The model under review builds one solid part; all positions refer to its coordinate system, in mm. Face numbers are marked on the shaded views. A direction names the side the tool comes from. Round coordinates to 2 decimals unless told otherwise and drop trailing zeros. Order: outer loops, then holes, each group sorted by start corner. A loop starts at its lowest first (then second) coordinate and runs counter-clockwise, first axis right, second up. Notation, with made-up numbers: M 83.5,-38 L 137.5,-38 A20 cw 137.5,-3 Z; hole C 72,57.25 d1. An arc over 180 degrees is marked long. Answer as CSV lines item,"result". Start each with the question number.
from build123d import *

# Parameters (mm, degrees)
F0_W     = 13
F0_H     = 13
F1_DEPTH = 70
F2_R     = 2
F3_R     = 5.25
F4_DEPTH = 30


with BuildPart() as f1:
    # F0 (on Top) → F1 (new body)
    with BuildSketch(Plane.XY):
        Rectangle(F0_W, F0_H)
    extrude(amount=F1_DEPTH)

    # F2
    f2_edges = [f1.edges().sort_by_distance(p)[0] for p in [
        (0, 6.5, 70),
        (-6.5, 0, 70),
        (0, -6.5, 70),
        (6.5, 0, 70),
    ]]
    fillet(f2_edges, radius=F2_R)

    # F3 (on face) → F4 (join)
    with BuildSketch(Plane.XZ.offset(6.5)):
        with Locations((0, 61.068749)):
            Circle(F3_R)
    extrude(amount=F4_DEPTH)


solid = f1.part
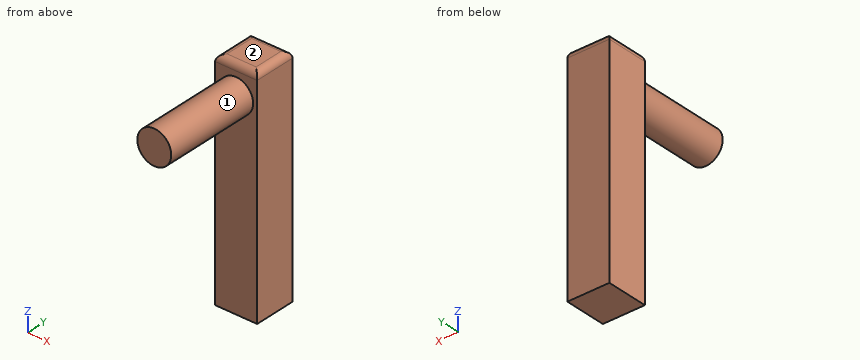
Item 1: Tool access review of the marked faces 1 and 2: name each direction out of +Z, -Z, +X, -X, +Y, -Y from which nothing blocks a thin tool from reaching the whole face with its end or side.
Item 2: Consider section C-C (y = -24.5). State the section outline as (x, z) points, and give its area (3 significant figures).
Item 3: Wall thickness on probe 1 along Y at (x, z) = (3.75, 54.5); probe 2 along Z at (x, y) = (4.75, 0); probe 3 along Z at (x, y) = (5.25, 2): over which ranges is each line inside the solid? List them lowest first. Write a range as [from, to].
Item 4: Consider section A-A (x = 0). State the section outline as (y, z) points, and give its area (3 significant figures).
Item 5: For pin 1 (1.5 mm diameter, centred on x = 0.5, y = -12, fed in from -Z); pin 2 (4 mm diameter, centred on x = 0, z = 37, fed in from -Y); pin 3 (10 mm diameter, centred on y = -10.5, z = 28.5, fed in from +X); pin 4 (4 mm diameter, centred on y = -9.5, z = 62.5, fed in from -X), all flat-tipped, find the tip position at first contact; note any pin that passes through.
Item 6: Consider section B-B (z = 5). State the section outline as (x, y) points, and give its area (3 significant figures).
Reported:
1,face 1,"-Y"
1,face 2,"+Z, +X, -X, +Y, -Y"
2,outline,"C 0,61.07 d10.5"
2,area,"86.6 mm²"
3,probe 1,"y = [-6.5, 6.5]"
3,probe 2,"z = [0, 69.98]"
3,probe 3,"z = [0, 69.85]"
4,outline,"M -36.5,55.82 L -6.5,55.82 L -6.5,0 L 6.5,0 L 6.5,68 A2 ccw 4.5,70 L -4.5,70 A2 ccw -6.5,68 L -6.5,66.32 L -36.5,66.32 Z"
4,area,"1,220 mm²"
5,pin 1,"stops at z = 55.82"
5,pin 2,"stops at y = -6.5"
5,pin 3,"stops at x = 6.5"
5,pin 4,"stops at x = -5.25"
6,outline,"M -6.5,-6.5 L 6.5,-6.5 L 6.5,6.5 L -6.5,6.5 Z"
6,area,"169 mm²"
